Geometry: final body of the model. Coordinates: model frame, mm. A direction names the side the tool comes from. Give positions to 0.01 mm unless a question says otherwise; leave off trailing zeros. Write each loop counter-clockwise with the first axis right and the second up, starting at its lowest first coordinate (ties: lowest second). Pieces come first, ordered by that corner, then holes. Notation, with made-up numbers: (-7.5, -23.75) - (31.5, -23.75) arc R17 cw to (31.5, -12.75) - close; hole circle Ø3 at (75, 55). An arc over 180 degrees is marked (long way). Return JSON: item names as keys, results as strings.
from build123d import *

# Parameters (mm, degrees)
SKETCH_1_R          = 1.75
SKETCH_1_R_2        = 1.5
EXTRUDE_1_DEPTH     = 9
FILLET_1_R          = 5
CUT_EXTRUDE_1_DEPTH = 3.5
SKETCH_5_R          = 3.75
CUT_EXTRUDE_2_DEPTH = 5
FILLET_2_R          = 2


with BuildPart() as part:
    # 草图1 → 凸台-拉伸1 (new body)
    with BuildSketch(Plane.XY):
        Polygon((-27.555241702, 0), (27.555241702, 0), (56.53301649, -7.764571353), (52.366592329, -23.31387801), (33.048075803, -18.137497108), (30.459885352, -27.796755371), (49.778401878, -32.973136273), (45.611977716, -48.52244293), (16.634202927, -40.757871577), (-16.634202927, -40.757871577), (-45.611977716, -48.52244293), (-49.778401878, -32.973136273), (-30.459885352, -27.796755371), (-33.048075803, -18.137497108), (-52.366592329, -23.31387801), (-56.53301649, -7.764571353), align=None)
        with Locations((-26.282483038, -4.75)):
            Circle(SKETCH_1_R, mode=Mode.SUBTRACT)
        with Locations((-17.863593392, -36.169723902)):
            Circle(SKETCH_1_R, mode=Mode.SUBTRACT)
        with Locations((17.863593392, -36.169723902)):
            Circle(SKETCH_1_R, mode=Mode.SUBTRACT)
        with Locations((26.282483038, -4.75)):
            Circle(SKETCH_1_R, mode=Mode.SUBTRACT)
        with Locations((-45.482028723, -15.257507669)):
            Circle(SKETCH_1_R_2, mode=Mode.SUBTRACT)
        with Locations((-22.350576875, -20.447491811)):
            Circle(SKETCH_1_R_2, mode=Mode.SUBTRACT)
        with Locations((-39.788009731, -36.507875848)):
            Circle(SKETCH_1_R_2, mode=Mode.SUBTRACT)
        with Locations((45.482028723, -15.257507669)):
            Circle(SKETCH_1_R_2, mode=Mode.SUBTRACT)
        with Locations((39.788009731, -36.507875848)):
            Circle(SKETCH_1_R_2, mode=Mode.SUBTRACT)
        with Locations((22.350576875, -20.447491811)):
            Circle(SKETCH_1_R_2, mode=Mode.SUBTRACT)
    extrude(amount=EXTRUDE_1_DEPTH)

    # 圆角1
    fillet_1_edges = [part.edges().sort_by_distance(p)[0] for p in [
        (-45.611977716, -48.52244293, 4.5),
        (-56.53301649, -7.764571353, 4.5),
        (-27.555241702, 0, 4.5),
        (27.555241702, 0, 4.5),
        (56.53301649, -7.764571353, 4.5),
        (45.611977716, -48.52244293, 4.5),
        (16.634202927, -40.757871577, 4.5),
        (-16.634202927, -40.757871577, 4.5),
    ]]
    fillet(fillet_1_edges, radius=FILLET_1_R)

    # 草图2 → 切除-拉伸1 (cut)
    with BuildSketch(Plane(origin=(0, 0, 0), x_dir=(-1, 0, 0), z_dir=(0, 0, -1))):
        Polygon((-42.303266769, -14.405760971), (-44.630282024, -12.078745715), (-47.809043978, -12.930492414), (-48.660790677, -16.109254368), (-46.333775421, -18.436269623), (-43.155013467, -17.584522925), align=None)
        Polygon((-21.498830176, -23.626253766), (-19.17181492, -21.29923851), (-20.023561619, -18.120476556), (-23.202323573, -17.268729857), (-25.529338829, -19.595745113), (-24.67759213, -22.774507067), align=None)
        Polygon((-36.609247776, -35.656129149), (-38.936263032, -33.329113893), (-42.115024986, -34.180860592), (-42.966771685, -37.359622546), (-40.639756429, -39.686637802), (-37.460994475, -38.834891103), align=None)
        Polygon((37.460994475, -38.834891103), (36.609247776, -35.656129149), (38.936263032, -33.329113893), (42.115024986, -34.180860592), (42.966771685, -37.359622546), (40.639756429, -39.686637802), align=None)
        Polygon((43.155013467, -17.584522925), (42.303266769, -14.405760971), (44.630282024, -12.078745715), (47.809043978, -12.930492414), (48.660790677, -16.109254368), (46.333775421, -18.436269623), align=None)
        Polygon((24.67759213, -22.774507067), (21.498830176, -23.626253766), (19.17181492, -21.29923851), (20.023561619, -18.120476556), (23.202323573, -17.268729857), (25.529338829, -19.595745113), align=None)
    extrude(amount=-CUT_EXTRUDE_1_DEPTH, mode=Mode.SUBTRACT)

    # 草图5 → 切除-拉伸2 (cut)
    with BuildSketch(Plane.XY.offset(9)):
        with Locations((-26.282483038, -4.75)):
            Circle(SKETCH_5_R)
        with Locations((-17.863593392, -36.169723902)):
            Circle(SKETCH_5_R)
        with Locations((17.863593392, -36.169723902)):
            Circle(SKETCH_5_R)
        with Locations((26.282483038, -4.75)):
            Circle(SKETCH_5_R)
    extrude(amount=-CUT_EXTRUDE_2_DEPTH, mode=Mode.SUBTRACT)

    # 圆角2
    fillet_2_edges = [part.edges().sort_by_distance(p)[0] for p in [
        (-49.778401878, -32.973136273, 4.5),
        (-30.459885352, -27.796755371, 4.5),
        (-33.048075803, -18.137497108, 4.5),
        (-52.366592329, -23.31387801, 4.5),
        (52.366592329, -23.31387801, 4.5),
        (33.048075803, -18.137497108, 4.5),
        (30.459885352, -27.796755371, 4.5),
        (49.778401878, -32.973136273, 4.5),
    ]]
    fillet(fillet_2_edges, radius=FILLET_2_R)


solid = part.part
Q1. Section query A-A, the plane y = -4.75. Return the cut outline in (x, z).
Answer key:
{"outline": "(-45.28, 0) - (-28.03, 0) - (-28.03, 4) - (-30.03, 4) - (-30.03, 9) - (-45.28, 9) - close; (-24.53, 0) - (24.53, 0) - (24.53, 4) - (22.53, 4) - (22.53, 9) - (-22.53, 9) - (-22.53, 4) - (-24.53, 4) - close; (28.03, 0) - (45.28, 0) - (45.28, 9) - (30.03, 9) - (30.03, 4) - (28.03, 4) - close"}
Q2. Section query D-D, the plane z = 1.75. Count the separate pieces of the cut face and the enclosed holes in it, plus the area to 3 significant figures.
Answer key:
{"separate pieces": "1", "enclosed holes": "10", "area": "3,700 mm^2"}
Q3. Section query B-B, the plane y = -42. Return the cut outline in (x, z).
Answer key:
{"outline": "(-47.36, 0) - (-21.27, 0) - (-21.27, 9) - (-47.36, 9) - close; (21.27, 0) - (47.36, 0) - (47.36, 9) - (21.27, 9) - close"}
Q4. Mould query, pull axis Y, two halves, no side actions, for faces 4 (the flat face through (-40.5, -33.75, 1.73)), 5 (the flat face through (-28.862, -44.034, 4.437)), 6 (the cylindrical face through (-54.71, -8.75, 4.56)). Classes: pulls with the +Y half, pulls with the -Y half, needs draft (parallel to the pull), parting line crosses it, or undercut.
Answer key:
{"face 4": "undercut", "face 5": "pulls with the -Y half", "face 6": "parting line crosses it"}
Q5. Section query C-C, the plane x = -1. Return the cut outline in (y, z).
Answer key:
{"outline": "(-40.76, 0) - (0, 0) - (0, 9) - (-40.76, 9) - close"}
Q6. Material intervals for probe 1 along X at (y, z) = (-7, 5.5); probe 2 along Y at (x, z) = (-16.5, 1.5); probe 3 along Y at (x, z) = (-21, 5), sorted ascending. Write a range as [from, to].
Answer key:
{"probe 1": "x = [-52.96, -29.28], [-23.28, 23.28], [29.28, 52.96]", "probe 2": "y = [-40.79, -37.27], [-35.07, 0]", "probe 3": "y = [-41.93, -38.23], [-34.11, -21.1], [-19.79, 0]"}
Q7. Pin query (flat end, axial travel): P1, Ø7, axis at x = -17.86, y = -36.17, coming from the +Z side; P2, Ø5, axis at x = -39.79, y = -36.51, coming from the -Z side; P3, Ø5, axis at x = 19, z = 3, coming from the -Y side. Return the tip coordinate at first contact, or that it passes through.
Answer key:
{"P1": "stops at z = 4", "P2": "stops at z = 3.5", "P3": "stops at y = -42.06"}
Q8. Set-up query: faces 1 (the cylindrical face through (15.1, -33.635, 6.535)), 2 (the cylindrical face through (43.983, -15.192, 6.212)), 3 (the flat face through (-42.535, -35.748, 1.726)). Return all of +Z, -Z, +X, -X, +Y, -Y with unobstructed straight access to the full face (end or side cutting, diameter ignored); none if empty.
Answer key:
{"face 1": "+Z", "face 2": "+Z, -Z", "face 3": "-Z"}
